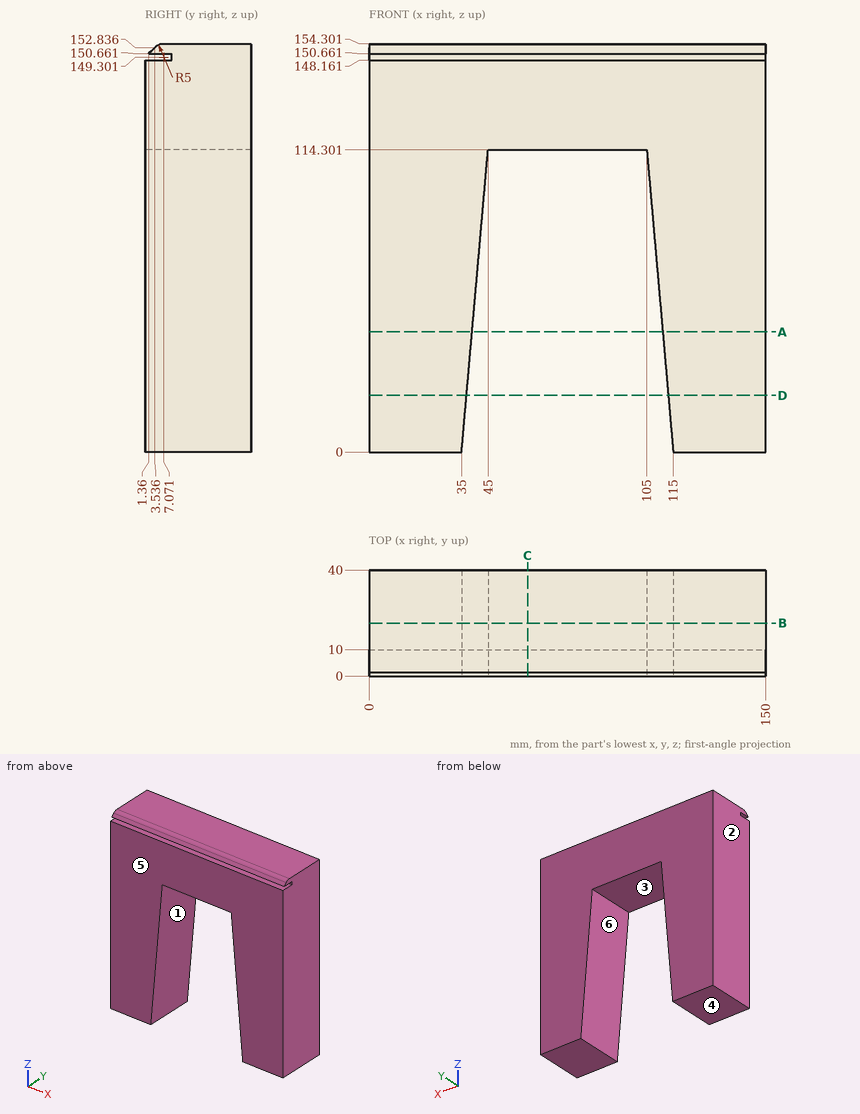
Can you work these out from the drawing? Everything is in mm from the part's minimum corner. A direction names the side the tool comes from. Coordinates: 2 decimals unless noted, no trailing zeros. Order: outer loops, then holes, each group sorted by start corner. A loop starts at its lowest first (then second) coordinate and runs counter-clockwise, first axis right, second up. Notation, with made-up numbers: (48, 46.5) -> (100, 46.5) arc R21 ccw to (100, 65.5) -> close; hole circle Ø10 at (-7, -35). An arc over 180 degrees is marked (long way). Return JSON: item names as keys, results as strings.
1) Thinking about a two-plate mould opening in X: for the marked faces 1, 2, 3 and 4, which applies, +X half, -X half, draft (parallel to the pull), parting line (faces both ways), or undercut?
Conclusion:
{"face 1": "undercut", "face 2": "-X half", "face 3": "undercut", "face 4": "draft"}
2) If I drill on probe 1 along Z at (x, y) = (129, 9); probe 2 along Z at (x, y) = (53, 12); probe 3 along X at (y, z) = (28.5, 106), over which ranges is the centre line in solid material (lowest first)?
Conclusion:
{"probe 1": "z = 0 to 148.16, 150.66 to 154.3", "probe 2": "z = 114.3 to 154.3", "probe 3": "x = 0 to 44.27, 105.73 to 150"}
3) On a 3-axis mill with a long thin cutter (end or side, diameter ignored), from which of +Z, -Z, +X, -X, +Y, -Y can I reach the whole of each face in a straight line? I mean the marked faces 5 and 6. Say none if no direction works.
Conclusion:
{"face 5": "+Z, -Z, +X, -X, -Y", "face 6": "-Z, +Y, -Y"}
4) If we section it at A-A on z = 45.5: List the corners of the cut face in (x, y) for me, plus the area to 3 significant figures.
Conclusion:
{"outline": "(0, 0) -> (38.98, 0) -> (38.98, 40) -> (0, 40) -> close; (111.02, 0) -> (150, 0) -> (150, 40) -> (111.02, 40) -> close", "area": "3,120 mm²"}
5) If we section it at D-D on z = 21.5: List the corners of the cut face in (x, y) for me, plus the area to 3 significant figures.
Conclusion:
{"outline": "(0, 0) -> (36.88, 0) -> (36.88, 40) -> (0, 40) -> close; (113.12, 0) -> (150, 0) -> (150, 40) -> (113.12, 40) -> close", "area": "2,950 mm²"}
6) If we section it at B-B on y = 20: List the corners of the cut face in (x, z) for me, plus the area to 3 significant figures.
Conclusion:
{"outline": "(0, 0) -> (35, 0) -> (45, 114.3) -> (105, 114.3) -> (115, 0) -> (150, 0) -> (150, 154.3) -> (0, 154.3) -> close", "area": "15,100 mm²"}
7) If we section it at C-C on x = 60: List the corners of the cut face in (y, z) for me (1 decimal), plus the area to 3 significant figures.
Conclusion:
{"outline": "(0, 114.3) -> (40, 114.3) -> (40, 154.3) -> (7.1, 154.3) arc R5 ccw to (3.5, 152.8) -> (1.4, 150.7) -> (10, 150.7) -> (10, 148.2) -> (0, 148.2) -> close", "area": "1,560 mm²"}
8) I'm going to push flat-ended pins straight in: P1, Ø6, axis at x = 91, y = 25.5, coming from the -Z side; P2, Ø2, axis at x = 46, z = 149, coming from the -Y side. Where does each tip first touch, or does it pass through?
Conclusion:
{"P1": "stops at z = 114.3", "P2": "stops at y = 0"}
